Geometry: final body of the model. Coordinates: model frame, mm. A direction names the side the tool comes from. Give positions to 0.01 mm unless a question says otherwise; leave off trailing zeros. Write each loop counter-clockwise with the first axis right and the second up, starting at its lowest first coordinate (ties: lowest second). Pieces come first, ordered by that corner, then holes.
Q1. Draft query along X for faces 1 (the face through (9.54, 3, -0.61)), 2 (the face through (6.82, -1.13, -0.59)), 3 (the face through (1.588, 5, 0)). Return one class per face: pulls with the +X half, pulls with the -X half, needs draft (parallel to the pull), parting line crosses it, or undercut.
Q2. Cut plane B-B on z = -0.05. Return the cut outline in (x, y), plus the area to 3 significant figures.
Q3. Line query: L1, parallel to Z at x = 7.5, y = 0 (3 decimals); L2, parallel to Y at x = -5.5, z = 0 (3 decimals); L3, parallel to Y at x = 5.5, z = -1.1. Output: solid intervals per line, ascending.
Q4. Pin query (flat end, axial travel): pin 1 (1.1 mm diameter, centred on y = 6, z = 1, fed in from -X); pin 2 (1 mm diameter, centred on x = -4, z = -1.5, fed in from -Y); pin 3 (2 mm diameter, centred on y = 6.5, z = 0, fed in from +X). Return the tip coordinate at first contact, or that it passes through.
Q5. Reachability of faces 4 (the face through (3.824, 0.938, 1.146)), 5 (the face through (2, -4, 2.5)) from +Z, -Z, +X, -X, +Y, -Y: full face, straight path, thin tool, end or side. Return the list, or none.
Q6. Cut plane A-A on x = 0. Return the cut outline in (y, z).
```python
from build123d import *

# Parameters (mm, degrees)
SKETCH1_R               = 10
BOSS_EXTRUDE1_DEPTH     = 2.5
SKETCH4_R               = 1.275
CUT_EXTRUDE1_DEPTH      = 11
CUT_EXTRUDE1_DEPTH_BACK = 11
FILLET1_R               = 1.27


with BuildPart() as part:
    # Sketch1 → Boss-Extrude1 (new body, symmetric)
    with BuildSketch(Plane.XY):
        Circle(SKETCH1_R)
        with BuildLine():
            Line((1.5875, 3.60275072), (1.5875, 7.112))
            Line((1.5875, 7.112), (-1.5875, 7.112))
            Line((-1.5875, 7.112), (-1.5875, 3.60275072))
            ThreePointArc((-1.5875, 3.60275072), (-3.937, 0), (-1.5875, -3.60275072))
            Line((-1.5875, -3.60275072), (-1.5875, -7.112))
            Line((-1.5875, -7.112), (1.5875, -7.112))
            Line((1.5875, -7.112), (1.5875, -3.60275072))
            ThreePointArc((1.5875, -3.60275072), (3.937, 0), (1.5875, 3.60275072))
        make_face(mode=Mode.SUBTRACT)
    extrude(amount=BOSS_EXTRUDE1_DEPTH, both=True)

    # Sketch4 → Cut-Extrude1 (cut, two sides)
    with BuildSketch(Plane(origin=(0, 0, 0), x_dir=(0, 0, -1), z_dir=(1, 0, 0))) as cut_extrude1_sk:
        Circle(SKETCH4_R)
    extrude(amount=CUT_EXTRUDE1_DEPTH, mode=Mode.SUBTRACT)
    extrude(cut_extrude1_sk.sketch, amount=-CUT_EXTRUDE1_DEPTH_BACK, mode=Mode.SUBTRACT)

    # Fillet1
    fillet1_edges = [part.edges().sort_by_distance(p)[0] for p in [
        (-10, 0, 2.5),
    ]]
    fillet(fillet1_edges, radius=FILLET1_R)


solid = part.part
```
Data:
1. face 1: parting line crosses it
1. face 2: needs draft
1. face 3: undercut
2. outline: (-9.92, -1.27) arc R10 ccw to (9.92, -1.27) - (3.73, -1.27) arc R3.94 cw to (1.59, -3.6) - (1.59, -7.11) - (-1.59, -7.11) - (-1.59, -3.6) arc R3.94 cw to (-3.73, -1.27) - close; (-9.92, 1.27) - (-3.73, 1.27) arc R3.94 cw to (-1.59, 3.6) - (-1.59, 7.11) - (1.59, 7.11) - (1.59, 3.6) arc R3.94 cw to (3.73, 1.27) - (9.92, 1.27) arc R10 ccw to start
2. area: 213 mm2
3. L1: z = -2.5 to -1.275, 1.275 to 2.5
3. L2: y = -8.352 to -1.275, 1.275 to 8.352
3. L3: y = -8.35 to -0.64, 0.64 to 8.35
4. pin 1: stops at x = -8.38
4. pin 2: stops at y = -9.37
4. pin 3: stops at x = 8.35
5. face 4: +Z, -Z
5. face 5: +Z, +X, -X, +Y, -Y
6. outline: (-10, -2.5) - (-7.11, -2.5) - (-7.11, 2.5) - (-8.73, 2.5) arc R1.27 ccw to (-10, 1.23) - close; (7.11, -2.5) - (10, -2.5) - (10, 1.23) arc R1.27 ccw to (8.73, 2.5) - (7.11, 2.5) - close
